```python
from build123d import *

# Parameters (mm, degrees)
F1_DEPTH  = 80
F3_DEPTH  = 75
F5_DEPTH  = 80
F7_DEPTH  = 80
F9_W      = 115.3811365366
F9_H      = 141.341894865
F10_DEPTH = 97.9
F11_R     = 5
F12_R     = 1


with BuildPart() as f1:
    # F0 (on Top) → F1 (new body)
    with BuildSketch(Plane.XY):
        Polygon((-41.2332489645, 39.6297108009), (-54.2332489645, 39.6297108009), (-54.2332489645, -40.3702891991), (25.7667510355, -40.3702891991), (25.7667510355, -27.3702891991), (-41.2332489645, -27.3702891991), align=None)
    extrude(amount=-F1_DEPTH)

    # F2 (on face) → F3 (cut)
    with BuildSketch(Plane.XY):
        Polygon((-44.2332489645, 39.6297108009), (-51.2332489645, 39.6297108009), (-51.2332489645, -37.3702891991), (25.7667510355, -37.3702891991), (25.7667510355, -30.3702891991), (-44.2332489645, -30.3702891991), align=None)
    extrude(amount=-F3_DEPTH, mode=Mode.SUBTRACT)

    # F4 (on face) → F5 (join)
    with BuildSketch(Plane.YZ.offset(25.7667510355)):
        Polygon((-27.3702891991, -80), (-40.3702891991, -80), (-40.3702891991, -97), (9.6297108009, -97), (9.6297108009, -90), (-35.3702891991, -90), (-35.3702891991, -83), (-20.3702891991, -83), (-20.3702891991, -80), align=None)
    extrude(amount=-F5_DEPTH)

    # F6 (on face) → F7 (join)
    with BuildSketch(Plane(origin=(0, 39.6297108009, 0), x_dir=(-1, 0, 0), z_dir=(0, 1, 0))):
        Polygon((54.2332489645, -80), (34.2332489645, -80), (34.2332489645, -83), (49.2332489645, -83), (49.2332489645, -90), (5.3266771138, -90), (5.3266771138, -97), (41.2332489645, -97), (54.2332489645, -97), align=None)
    extrude(amount=-F7_DEPTH)

    # F9 (on offset) → F10 (cut)
    with BuildSketch(Plane(origin=(0, 0, -83), x_dir=(1, 0, 0), z_dir=(0, 0, -1))):
        with Locations((-4.7438181937, -3.1282007694)):
            Rectangle(F9_W, F9_H)
    extrude(amount=-F10_DEPTH, mode=Mode.SUBTRACT)

    # F11
    f11_edges = [f1.edges().sort_by_distance(p)[0] for p in [
        (-5.326677, 9.629711, -93.5),
        (-5.326677, 39.629711, -93.5),
        (25.766751, 9.629711, -93.5),
    ]]
    fillet(f11_edges, radius=F11_R)

    # F12
    f12_edges = [f1.edges().sort_by_distance(p)[0] for p in [
        (25.766751, -40.370289, -90),
        (-54.233249, 39.629711, -90),
    ]]
    fillet(f12_edges, radius=F12_R)


solid = f1.part
```
Geometry: final body of the model. Coordinates: model frame, mm. A direction names the side the tool comes from. Round coordinates to 2 decimals unless told otherwise and drop trailing zeros. Order: outer loops, then holes, each group sorted by start corner. A loop starts at its lowest first (then second) coordinate and runs counter-clockwise, first axis right, second up. Notation, with made-up numbers: (4, 31.5) -> (32, 31.5) arc R8 ccw to (32, 43.5) -> close; hole circle Ø3 at (-17, 12.25). An arc over 180 degrees is marked (long way). Use CSV: the item, a comma, the result in double quotes. Start each with the question number.
1) Section C-C (y = 23.5). Return the cut outline in (x, z), and give its area (3 significant figures).
2) Section B-B (x = 9). Return the cut outline in (y, z).
3) Material intervals for line 1 along Z through (x, y) = (-30.5, 19); line 2 along X through (y, z) = (-27, -83.5); line 3 along Y through (x, z) = (-8, -87.75), sorted ascending. Write a range as from..to.
4) Set-up query: faces 1 (the face through (-49.233, 3, -86)), 2 (the face through (10, 9.63, -94)), 3 (the face through (-31, 39.63, -93)). Return all of +Z, -Z, +X, -X, +Y, -Y with unobstructed straight access to the full face (end or side cutting, diameter ignored); none if empty.
5) First-contact query: pin 1 Ø7.5 at (y, z) = (20.5, -94.5) entering from +X; pin 2 Ø2 at (x, z) = (-6.5, -86) entering from +Y; pin 3 Ø2 at (x, z) = (13.5, -94.5) entering from +Y. Flat tips, straight axial feed; report the tip coordinate or a pass-through.
6) Section D-D (z = -85.25). Return the cut outline in (x, y), and give its area (3 significant figures).
7) Section A-A (z = -93.75). Return the cut outline in (x, y).
Returned:
1,outline,"(-54.23, -97) -> (-5.33, -97) -> (-5.33, -90) -> (-49.23, -90) -> (-49.23, -83) -> (-54.23, -83) -> close"
1,area,"377 mm²"
2,outline,"(-40.37, -97) -> (9.63, -97) -> (9.63, -90) -> (-35.37, -90) -> (-35.37, -83) -> (-40.37, -83) -> close"
3,line 1,"z = -97..-90"
3,line 2,"x = -54.23..-49.23"
3,line 3,"y = -40.37..-35.37"
4,face 1,"+Z, +X, +Y"
4,face 2,"+Z, -Z, +X, +Y"
4,face 3,"+Z, -Z, +X, -X, +Y"
5,pin 1,"stops at x = -5.33"
5,pin 2,"stops at y = -35.37"
5,pin 3,"stops at y = 9.63"
6,outline,"(-54.23, -40.37) -> (24.77, -40.37) arc R1 ccw to (25.77, -39.37) -> (25.77, -35.37) -> (-49.23, -35.37) -> (-49.23, 39.63) -> (-53.23, 39.63) arc R1 ccw to (-54.23, 38.63) -> close"
6,area,"775 mm²"
7,outline,"(-54.23, -40.37) -> (24.77, -40.37) arc R1 ccw to (25.77, -39.37) -> (25.77, 4.63) arc R5 ccw to (20.77, 9.63) -> (-0.33, 9.63) arc R5 cw to (-5.33, 14.63) -> (-5.33, 34.63) arc R5 ccw to (-10.33, 39.63) -> (-53.23, 39.63) arc R1 ccw to (-54.23, 38.63) -> close"
